Part model, mm, in its own coordinate system. Round coordinates to 2 decimals unless told otherwise and drop trailing zeros. Write each loop counter-clockwise with the first axis right and the second up, starting at its lowest first coordinate (ties: lowest second). Pieces come first, ordered by that corner, then holes. Notation, with made-up numbers: M 78.5,67.25 L 134.5,67.25 A22 ccw 134.5,83.25 Z; hole C 47.25,59.5 d4. An arc over 180 degrees is marked long. Use one line per item in the form item = value. Start each with the question number.
Item 1: Probe L1, parallel to X at y = -36.5, z = 2.7; L2, parallel to Y at x = 47, z = 1.35; L3, parallel to Y at x = 15.5, z = 1.5. List the from-to ranges inside material, lowest first.
Item 2: Cut at A-A, the plane x = 54.5. Give the cut face in (y, z), then the cut area to 3 significant figures.
Item 3: Flat gauge pin, fed straight in: pin 1 Ø0.9 at (x, z) = (-64, 1.5) entering from +Y. Where does the tip first touch, or does it go through?
Item 4: Cut at C-C, the plane x = -51. Give the cut face in (y, z), then the cut area to 3 significant figures.
Item 5: Cut at B-B, the plane y = 52. Give the cut face in (x, z).
Item 6: Cut at D-D, the plane z = 1.15. State how many separate pieces and enclosed holes the cut face has, then the cut area to 3 significant figures.
from build123d import *

# Parameters (mm, degrees)
F0_R     = 1.9812
F0_R_2   = 1.3716
F0_W     = 4.99999
F0_H     = 51.988186
F0_W_2   = 17
F0_H_2   = 10.000005
F0_W_3   = 5.005598
F0_H_3   = 51.988198
F0_R_3   = 1.5
F1_DEPTH = 2.999994


with BuildPart() as f1:
    # F0 (on Top) → F1 (new body)
    with BuildSketch(Plane.XY):
        with BuildLine():
            ThreePointArc((-161.572698, -117.981502), (-160.412138, -120.783342), (-157.610298, -121.943902))
            Line((-157.610298, -121.943902), (139.264902, -121.943902))
            ThreePointArc((139.264902, -121.943902), (142.066742, -120.783342), (143.227302, -117.981502))
            Line((143.227302, -117.981502), (143.227302, 117.806698))
            ThreePointArc((143.227302, 117.806698), (142.066742, 120.608538), (139.264902, 121.769098))
            Line((139.264902, 121.769098), (-9.640698, 121.769098))
            ThreePointArc((-9.640698, 121.769098), (-12.442255, 120.608655), (-13.602698, 117.807098))
            Line((-13.602698, 117.807098), (-13.602698, 113.769098))
            Line((-13.602698, 113.769098), (-18.621498, 113.769098))
            Line((-18.621498, 113.769098), (-18.621498, 111.609098))
            ThreePointArc((-18.621498, 111.609098), (-20.602698, 109.627898), (-22.583898, 111.609098))
            Line((-22.583898, 111.609098), (-22.583898, 113.769098))
            Line((-22.583898, 113.769098), (-143.081498, 113.769098))
            Line((-143.081498, 113.769098), (-143.081498, 111.609098))
            ThreePointArc((-143.081498, 111.609098), (-145.062698, 109.627898), (-147.043898, 111.609098))
            Line((-147.043898, 111.609098), (-147.043898, 113.769098))
            Line((-147.043898, 113.769098), (-157.610698, 113.769098))
            ThreePointArc((-157.610698, 113.769098), (-160.412255, 112.608655), (-161.572698, 109.807098))
            Line((-161.572698, 109.807098), (-161.572698, -117.981502))
        make_face()
        with Locations((-145.062698, -115.720902)):
            Circle(F0_R, mode=Mode.SUBTRACT)
        with Locations((-126.572768, -91.248119)):
            Circle(F0_R_2, mode=Mode.SUBTRACT)
        with Locations((-20.602698, -115.720902)):
            Circle(F0_R, mode=Mode.SUBTRACT)
        with Locations((-77.576168, -91.248119)):
            Circle(F0_R_2, mode=Mode.SUBTRACT)
        with Locations((-71.023698, -62.253998)):
            Rectangle(F0_W, F0_H, mode=Mode.SUBTRACT)
        with Locations((-39.071038, -91.123914)):
            Circle(F0_R_2, mode=Mode.SUBTRACT)
        with Locations((-145.062698, -43.330902)):
            Circle(F0_R, mode=Mode.SUBTRACT)
        with Locations((-126.572768, -33.259919)):
            Circle(F0_R_2, mode=Mode.SUBTRACT)
        with Locations((-120.213727, -24.750785)):
            Rectangle(F0_W_2, F0_H_2, mode=Mode.SUBTRACT)
        with Locations((-77.576168, -33.259919)):
            Circle(F0_R_2, mode=Mode.SUBTRACT)
        with Locations((-39.071038, -33.135714)):
            Circle(F0_R_2, mode=Mode.SUBTRACT)
        with Locations((-20.602698, -43.330902)):
            Circle(F0_R, mode=Mode.SUBTRACT)
        with Locations((-32.702081, -24.750785)):
            Rectangle(F0_W_2, F0_H_2, mode=Mode.SUBTRACT)
        with Locations((9.925562, -91.123914)):
            Circle(F0_R_2, mode=Mode.SUBTRACT)
        with Locations((16.478031, -62.253998)):
            Rectangle(F0_W, F0_H, mode=Mode.SUBTRACT)
        with Locations((48.430692, -91.109401)):
            Circle(F0_R_2, mode=Mode.SUBTRACT)
        with Locations((136.877302, -115.593902)):
            Circle(F0_R, mode=Mode.SUBTRACT)
        with Locations((97.427292, -91.109401)):
            Circle(F0_R_2, mode=Mode.SUBTRACT)
        with Locations((105.110925, -62.253998)):
            Rectangle(F0_W_3, F0_H, mode=Mode.SUBTRACT)
        with Locations((9.925562, -33.135714)):
            Circle(F0_R_2, mode=Mode.SUBTRACT)
        with Locations((48.430692, -33.121201)):
            Circle(F0_R_2, mode=Mode.SUBTRACT)
        with Locations((54.808345, -24.750786)):
            Rectangle(F0_W_2, F0_H_2, mode=Mode.SUBTRACT)
        with Locations((97.427292, -33.121201)):
            Circle(F0_R_2, mode=Mode.SUBTRACT)
        with Locations((136.877302, -43.203902)):
            Circle(F0_R, mode=Mode.SUBTRACT)
        with Locations((-126.572768, 13.791184)):
            Circle(F0_R_2, mode=Mode.SUBTRACT)
        with Locations((-77.576168, 13.791184)):
            Circle(F0_R_2, mode=Mode.SUBTRACT)
        with Locations((-39.071038, 13.746255)):
            Circle(F0_R_2, mode=Mode.SUBTRACT)
        with Locations((-71.023698, 42.785289)):
            Rectangle(F0_W, F0_H_3, mode=Mode.SUBTRACT)
        with Locations((-126.572768, 71.779384)):
            Circle(F0_R_2, mode=Mode.SUBTRACT)
        with Locations((-120.213727, 80.288516)):
            Rectangle(F0_W_2, F0_H_2, mode=Mode.SUBTRACT)
        with Locations((-156.572698, 101.769098)):
            Circle(F0_R_3, mode=Mode.SUBTRACT)
        with Locations((-77.576168, 71.779384)):
            Circle(F0_R_2, mode=Mode.SUBTRACT)
        with Locations((-39.071038, 71.734455)):
            Circle(F0_R_2, mode=Mode.SUBTRACT)
        with Locations((-32.70208, 80.288516)):
            Rectangle(F0_W_2, F0_H_2, mode=Mode.SUBTRACT)
        with Locations((9.925562, 13.746255)):
            Circle(F0_R_2, mode=Mode.SUBTRACT)
        with Locations((48.430692, 13.850588)):
            Circle(F0_R_2, mode=Mode.SUBTRACT)
        with Locations((16.478031, 42.785289)):
            Rectangle(F0_W, F0_H_3, mode=Mode.SUBTRACT)
        with Locations((97.427292, 13.850588)):
            Circle(F0_R_2, mode=Mode.SUBTRACT)
        with Locations((105.110925, 42.785289)):
            Rectangle(F0_W_3, F0_H_3, mode=Mode.SUBTRACT)
        with Locations((9.925562, 71.734455)):
            Circle(F0_R_2, mode=Mode.SUBTRACT)
        with Locations((48.430692, 71.838788)):
            Circle(F0_R_2, mode=Mode.SUBTRACT)
        with Locations((54.808346, 80.288516)):
            Rectangle(F0_W_2, F0_H_2, mode=Mode.SUBTRACT)
        with Locations((-5.602698, 111.609098)):
            Circle(F0_R_3, mode=Mode.SUBTRACT)
        with Locations((97.427292, 71.838788)):
            Circle(F0_R_2, mode=Mode.SUBTRACT)
        with Locations((136.877302, 88.749098)):
            Circle(F0_R, mode=Mode.SUBTRACT)
    extrude(amount=F1_DEPTH)


solid = f1.part
Model answer:
q1.L1 = -161.57 to -73.52, -68.52 to 13.98, 18.98 to 102.61, 107.61 to 143.23
q1.L2 = -121.94 to -29.75, -19.75 to 75.29, 85.29 to 121.77
q1.L3 = -121.94 to -88.25, -36.26 to 16.79, 68.78 to 121.77
q2.outline = M -121.94,0 L -29.75,0 L -29.75,3 L -121.94,3 Z; M -19.75,0 L 75.29,0 L 75.29,3 L -19.75,3 Z; M 85.29,0 L 121.77,0 L 121.77,3 L 85.29,3 Z
q2.area = 671 mm²
q3.pin_1 = 113.77
q4.outline = M -121.94,0 L 113.77,0 L 113.77,3 L -121.94,3 Z
q4.area = 707 mm²
q5.outline = M -161.57,0 L -73.52,0 L -73.52,3 L -161.57,3 Z; M -68.52,0 L 13.98,0 L 13.98,3 L -68.52,3 Z; M 18.98,0 L 102.61,0 L 102.61,3 L 18.98,3 Z; M 107.61,0 L 143.23,0 L 143.23,3 L 107.61,3 Z
q6.separate_pieces = 1
q6.enclosed_holes = 45
q6.area = 70,200 mm²
